Source: CAD feature listing. Evaluate the final solid. Frame: model axes, mm. A direction names the side the tool comes from. Give positions to 0.01 mm unless a question says otherwise; leave off trailing zeros. Loops run counter-clockwise (first coordinate to the right, second up) from the corner with the lowest first, then second, coordinate; pieces in that order, holes last. Notation, with made-up numbers: (-0.5, -25) -> (47.5, -25) arc R25 cw to (47.5, -5) -> close; hole circle Ø8 at (39, 78). An arc over 180 degrees is marked (long way). Put each result on its own line as item: value.
```python
from build123d import *

# Parameters (mm, degrees)
F0_R      = 37.5
F1_DEPTH  = 7
F2_R      = 35.5
F3_DEPTH  = 5
F4_SIZE   = 0.5
F6_DEPTH  = 3
F7_W      = 4
F7_H      = 5
F8_DEPTH  = 3
F9_W      = 4
F9_H      = 5
F10_DEPTH = 3
F12_DEPTH = 2


with BuildPart() as f1:
    # F0 (on Top) → F1 (new body)
    with BuildSketch(Plane.XY):
        Circle(F0_R)
    extrude(amount=F1_DEPTH)

    # F2 (on face) → F3 (cut)
    with BuildSketch(Plane.XY.offset(7)):
        Circle(F2_R)
    extrude(amount=-F3_DEPTH, mode=Mode.SUBTRACT)

    # F4
    f4_edges = [f1.edges().sort_by_distance(p)[0] for p in [
        (-37.5, 0, 7),
    ]]
    chamfer(f4_edges, length=F4_SIZE)

    # F5 (on face) → F6 (join)
    with BuildSketch(Plane(origin=(0, 0, 0), x_dir=(1, 0, 0), z_dir=(0, 0, -1))):
        with BuildLine():
            ThreePointArc((-17, 33.4252898267), (-8.740756017, 36.467097283), (0, 37.5))
            Line((0, 37.5), (0, 47.5))
            Line((0, 47.5), (-17, 47.5))
            Line((-17, 47.5), (-17, 33.4252898267))
        make_face()
        with BuildLine():
            Line((0, 47.5), (0, 37.5))
            ThreePointArc((0, 37.5), (8.740756017, 36.467097283), (17, 33.4252898267))
            Line((17, 33.4252898267), (17, 47.5))
            Line((17, 47.5), (0, 47.5))
        make_face()
        with BuildLine():
            Line((0, -47.5), (0, -37.5))
            ThreePointArc((0, -37.5), (-8.740756017, -36.467097283), (-17, -33.4252898267))
            Line((-17, -33.4252898267), (-17, -47.5))
            Line((-17, -47.5), (0, -47.5))
        make_face()
        with BuildLine():
            ThreePointArc((17, -33.4252898267), (8.740756017, -36.467097283), (0, -37.5))
            Line((0, -37.5), (0, -47.5))
            Line((0, -47.5), (17, -47.5))
            Line((17, -47.5), (17, -33.4252898267))
        make_face()
    extrude(amount=-F6_DEPTH)

    # F7 (on face) → F8 (cut, through all)
    with BuildSketch(Plane.XY.offset(3)):
        with BuildLine():
            Line((4, 42.5), (0, 42.5))
            Line((0, 42.5), (-4, 42.5))
            Line((-4, 42.5), (-12, 42.5))
            Line((-12, 42.5), (-12, 35.528157847))
            ThreePointArc((-12, 35.528157847), (0, 37.5), (12, 35.528157847))
            Line((12, 35.528157847), (12, 42.5))
            Line((12, 42.5), (4, 42.5))
        make_face()
        with Locations((2, 45)):
            Rectangle(F7_W, F7_H)
        with Locations((-2, 45)):
            Rectangle(F7_W, F7_H)
    extrude(amount=-F8_DEPTH, mode=Mode.SUBTRACT)

    # F9 (on face) → F10 (cut, through all)
    with BuildSketch(Plane.XY.offset(3)):
        with BuildLine():
            Line((-4, -42.5), (0, -42.5))
            Line((0, -42.5), (4, -42.5))
            Line((4, -42.5), (12, -42.5))
            Line((12, -42.5), (12, -35.528157847))
            ThreePointArc((12, -35.528157847), (0, -37.5), (-12, -35.528157847))
            Line((-12, -35.528157847), (-12, -42.5))
            Line((-12, -42.5), (-4, -42.5))
        make_face()
        with Locations((2, -45)):
            Rectangle(F9_W, F9_H)
        with Locations((-2, -45)):
            Rectangle(F9_W, F9_H)
    extrude(amount=-F10_DEPTH, mode=Mode.SUBTRACT)

    # F11 (on face) → F12 (cut, through all)
    with BuildSketch(Plane.XY.offset(2)):
        with BuildLine():
            Line((5, 5), (25.9183331907, 5))
            ThreePointArc((25.9183331907, 5), (18.6649403345, 18.6649403345), (5, 25.9183331907))
            Line((5, 25.9183331907), (5, 5))
        make_face()
        with BuildLine():
            Line((-5, 5), (-5, 25.9183331907))
            ThreePointArc((-5, 25.9183331907), (-18.6649403345, 18.6649403345), (-25.9183331907, 5))
            Line((-25.9183331907, 5), (-5, 5))
        make_face()
        with BuildLine():
            ThreePointArc((5, -25.9183331907), (18.6649403345, -18.6649403345), (25.9183331907, -5))
            Line((25.9183331907, -5), (5, -5))
            Line((5, -5), (5, -25.9183331907))
        make_face()
        with BuildLine():
            ThreePointArc((-25.9183331907, -5), (-18.6649403345, -18.6649403345), (-5, -25.9183331907))
            Line((-5, -25.9183331907), (-5, -5))
            Line((-5, -5), (-25.9183331907, -5))
        make_face()
    extrude(amount=-F12_DEPTH, mode=Mode.SUBTRACT)


solid = f1.part
```
(1) Section A-A on z = 4.75. Return loops of the section in (x, y).
Calculated:
outline: circle Ø75 at (0, 0); hole circle Ø71 at (0, 0)
(2) Reachability of faces 4 (the flat face through (-4, 45, 2)), 5 (the flat face through (-17, 40, 1)), 6 (the flat face through (17, -40, 1)), 7 (the cylindrical face through (-7.696, -34.656, 4.535)), 8 (the flat face through (12, 39, 2)) from +Z, -Z, +X, -X, +Y, -Y: full face, straight path, thin tool, end or side. Return the list, or none.
Calculated:
face 4: +Z, -Z, +Y
face 5: +Z, -Z, -X, +Y
face 6: +Z, -Z, +X, -Y
face 7: +Z
face 8: +Z, -Z
(3) Line query: probe 1 along X at (y, z) = (42, 1); probe 2 along Y at (x, z) = (0, 4.7); probe 3 along Z at (x, y) = (-25.5, 0). Output: solid intervals per line, ascending. Write a range as from..to.
Calculated:
probe 1: x = -17..-12, 12..17
probe 2: y = -37.5..-35.5, 35.5..37.5
probe 3: z = 0..2
(4) Draft query along Y for faces 1 (the flat face through (-11, 47.5, 1)), 2 (the flat face through (12, -44, 3)), 3 (the flat face through (12, -39, 2)). Return one class per face: released by +Y, released by -Y, zero draft, split by the parting line, or undercut.
Calculated:
face 1: released by +Y
face 2: zero draft
face 3: undercut
(5) Section D-D on y = -20.5. Give the number of separate pieces and of enclosed holes in the cut face, then the cut area to 3 significant figures.
Calculated:
separate pieces: 3
enclosed holes: 0
area: 103 mm²
(6) Section B-B on x = 0. Return loops of the section in (y, z).
Calculated:
outline: (-37.5, 0) -> (37.5, 0) -> (37.5, 6.5) -> (37, 7) -> (35.5, 7) -> (35.5, 2) -> (-35.5, 2) -> (-35.5, 7) -> (-37, 7) -> (-37.5, 6.5) -> close
(7) First-contact query: P1, Ø1.6, axis at x = -19, z = 1.5, coming from the +Y side; P2, Ø0.9, axis at y = -40, z = 1.5, coming from the +X side; P3, Ø4, axis at y = -29, z = 2, coming from the +X side. Flat tips, straight axial feed; report the tip coordinate or a pass-through.
Calculated:
P1: stops at y = 32.79
P2: stops at x = 17
P3: stops at x = 26.02
